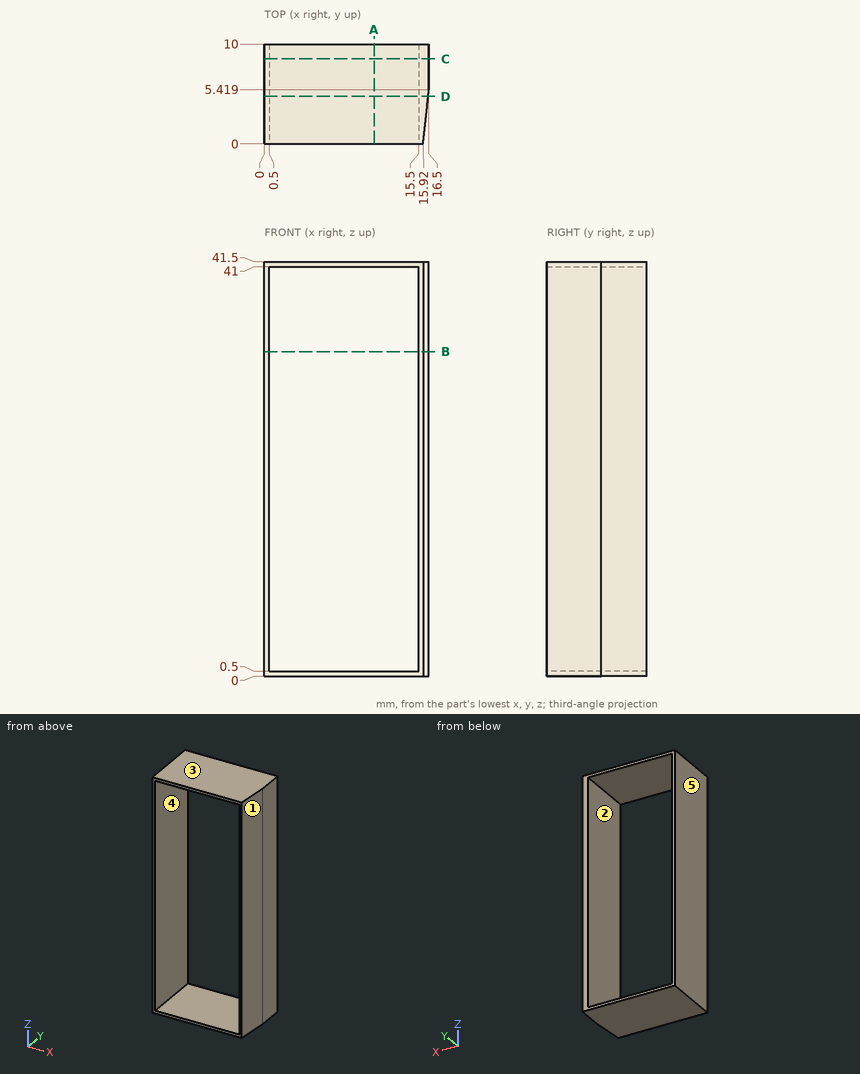
Drawing for the job (mm, zero at the part's lowest x, y, z). A direction names the side the tool comes from. Give positions to 0.01 mm unless a question says otherwise; leave off trailing zeros. Loops run counter-clockwise (first coordinate to the right, second up) from the corner with the lowest first, then second, coordinate; pieces in that order, holes last.
Item 1: Slice it at C-C (y = 8.5). Write the cut outline in (x, z).
Check values:
outline: (0, 0) - (16.5, 0) - (16.5, 41.5) - (0, 41.5) - close; hole (0.5, 0.5) - (15.5, 0.5) - (15.5, 41) - (0.5, 41) - close
Item 2: Drill centre lines: line 1 along Z through (x, y) = (13.5, 9.25); line 2 along X through (y, z) = (9.75, 25.5); line 3 along X through (y, z) = (4.75, 36.5). Where is each one in solid material? Low to high.
Check values:
line 1: z = 0 to 0.5, 41 to 41.5
line 2: x = 0 to 0.5, 15.5 to 16.5
line 3: x = 0 to 0.5, 15.5 to 16.43
Item 3: Slice it at A-A (x = 11). Write the cut outline in (y, z), plus the area to 3 significant figures.
Check values:
outline: (0, 0) - (10, 0) - (10, 0.5) - (0, 0.5) - close; (0, 41) - (10, 41) - (10, 41.5) - (0, 41.5) - close
area: 10.0 mm2
Item 4: Slice it at D-D (y = 4.75). Write the cut outline in (x, z).
Check values:
outline: (0, 0) - (16.43, 0) - (16.43, 41.5) - (0, 41.5) - close; hole (0.5, 0.5) - (15.5, 0.5) - (15.5, 41) - (0.5, 41) - close
Item 5: Which spindle directions (+Z, -Z, +X, -X, +Y, -Y) get a long thin tool onto all of the face, cutting with end or side? Do the marked faces 1 and 2. Say none if no direction does.
Check values:
face 1: +Z, -Z, +X, -Y
face 2: +Y, -Y
Item 6: Drop flat-ended pins along their axis: P1, Ø1, axis at y = 9, z = 14, coming from the -X side; P2, Ø1.5, axis at y = 1.5, z = 25, coming from the +X side. Give the stop position or say it passes through.
Check values:
P1: stops at x = 0
P2: stops at x = 16.16
Item 7: Mould opens along X. For the marked faces 3, 4 and 5 say: +X half, -X half, draft (parallel to the pull), parting line (faces both ways), or undercut.
Check values:
face 3: draft
face 4: undercut
face 5: -X half
Item 8: Slice it at B-B (z = 32.5). Write the cut outline in (x, y).
Check values:
outline: (0, 0) - (0.5, 0) - (0.5, 10) - (0, 10) - close; (15.5, 0) - (15.92, 0) - (16.5, 5.42) - (16.5, 10) - (15.5, 10) - close
